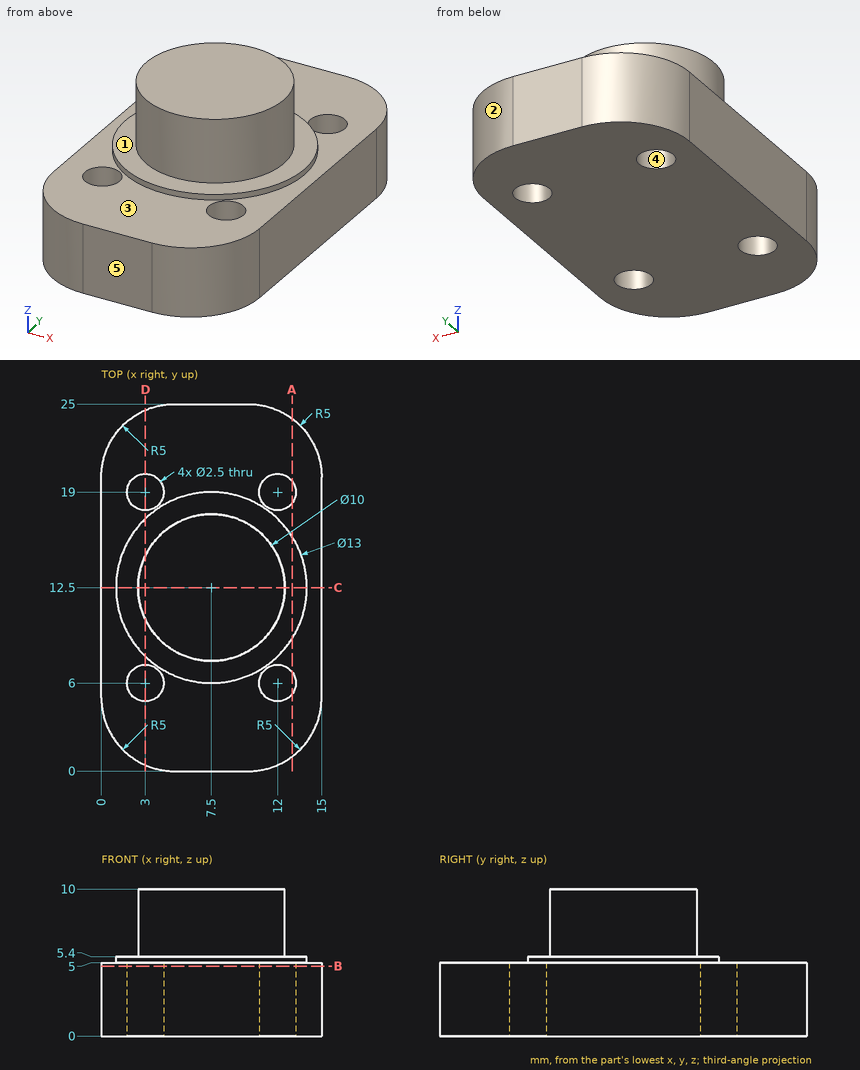
The drawing under review shows one solid part. Ordinate dimensions are in mm from its lowest x, y, z. A direction names the side the tool comes from. Round coordinates to 2 decimals unless told otherwise and drop trailing zeros. Loops run counter-clockwise (first coordinate to the right, second up) from the corner with the lowest first, then second, coordinate; pieces in that order, holes last. Notation, with made-up numbers: (0, 39.25) -> (8, 39.25) arc R19 cw to (8, 68.25) -> close; hole circle Ø8 at (16, -1.5). An arc over 180 degrees is marked (long way). One line per question, with ' | ' between items. Start each with the question number.
Item 1: Draft analysis for pull direction Y (two halves, no side actions). For the marked faces 3, 4 and 5, state which applies: +Y half, -Y half, draft (parallel to the pull), parting line (faces both ways), or undercut.
Item 2: Add section B-B, the plane z = 4.75. Write out the cut boundary in (x, y).
Item 3: Add section A-A, the plane x = 13. Write out the cut boundary in (y, z).
Item 4: Wall thickness on line 1 along X through (y, z) = (6.5, 1.75); line 2 along Y through (x, z) = (3, 3.15); line 3 along Z through (x, y) = (6, 1.5): over which ranges is each line inside the solid? List them lowest first. Write a range as [from, to].
Item 5: Add section D-D, the plane x = 3. Write out the cut boundary in (y, z).
Item 6: Add section C-C, the plane y = 12.5. Write out the cut boundary in (x, z), then the cut area to 3 significant figures.
Item 7: For pin 1 (2 mm diameter, centred on x = 3, y = 6, fed in from -Z); pin 2 (1 mm diameter, centred on x = 7, y = 10, fed in from -Z); pin 3 (3 mm diameter, centred on x = 13, z = 7, fed in from -Y); pin 4 (3 mm diameter, centred on x = 2.5, y = 5, fed in from +Z), all flat-tipped, find the tip position at first contact; note any pin that passes through.
Item 8: Machinability: for the marked faces 1 and 2, which of the approach directions +Z, -Z, +X, -X, +Y, -Y give a long, thin tool a straight path to every point of the face, cutting with its end or side? Answer none if there is none.
Return value:
1) face 3: draft | face 4: undercut | face 5: -Y half
2) outline: (0, 5) arc R5 ccw to (5, 0) -> (10, 0) arc R5 ccw to (15, 5) -> (15, 20) arc R5 ccw to (10, 25) -> (5, 25) arc R5 ccw to (0, 20) -> close; hole circle Ø2.5 at (3, 6); hole circle Ø2.5 at (3, 19); hole circle Ø2.5 at (12, 6); hole circle Ø2.5 at (12, 19)
3) outline: (1, 0) -> (5.25, 0) -> (5.25, 5) -> (1, 5) -> close; (6.75, 0) -> (18.25, 0) -> (18.25, 5) -> (15.96, 5) -> (15.96, 5.4) -> (9.04, 5.4) -> (9.04, 5) -> (6.75, 5) -> close; (19.75, 0) -> (24, 0) -> (24, 5) -> (19.75, 5) -> close
4) line 1: x = [0, 1.85], [4.15, 10.85], [13.15, 15] | line 2: y = [0.42, 4.75], [7.25, 17.75], [20.25, 24.58] | line 3: z = [0, 5]
5) outline: (0.42, 0) -> (4.75, 0) -> (4.75, 5) -> (0.42, 5) -> close; (7.25, 0) -> (17.75, 0) -> (17.75, 5) -> (17.19, 5) -> (17.19, 5.4) -> (14.68, 5.4) -> (14.68, 10) -> (10.32, 10) -> (10.32, 5.4) -> (7.81, 5.4) -> (7.81, 5) -> (7.25, 5) -> close; (20.25, 0) -> (24.58, 0) -> (24.58, 5) -> (20.25, 5) -> close
6) outline: (0, 0) -> (15, 0) -> (15, 5) -> (14, 5) -> (14, 5.4) -> (12.5, 5.4) -> (12.5, 10) -> (2.5, 10) -> (2.5, 5.4) -> (1, 5.4) -> (1, 5) -> (0, 5) -> close | area: 126 mm2
7) pin 1: passes through | pin 2: stops at z = 0 | pin 3: stops at y = 9.5 | pin 4: stops at z = 5
8) face 1: +Z | face 2: +Z, -Z, +X, +Y
